from build123d import *

# Parameters (mm, degrees)
CROQUIS1_R              = 4.75
CROQUIS1_R_2            = 3.275
SALIENTE_EXTRUIR1_DEPTH = 4.25
CROQUIS3_R              = 4.85
CROQUIS3_R_2            = 2.1
SALIENTE_EXTRUIR2_DEPTH = 2
REDONDEO1_R             = 0.6
REDONDEO2_R             = 1
CHAFL_N1_SIZE           = 0.7
CHAFL_N2_SIZE           = 0.5


with BuildPart() as part:
    # Croquis1 → Saliente-Extruir1 (new body)
    with BuildSketch(Plane(origin=(0, 0, 0), x_dir=(1, 0, 0), z_dir=(0, 1, 0))):
        Circle(CROQUIS1_R)
        Circle(CROQUIS1_R_2, mode=Mode.SUBTRACT)
    extrude(amount=SALIENTE_EXTRUIR1_DEPTH)

    # Croquis2 → Revolución1 (revolve)
    with BuildSketch(Plane.XY):
        Polygon((-4.75, 4.25), (-4.85, 5.25), (-2.1, 5.25), (-2.1, 5.15), (-3.275, 4.25), align=None)
    revolve(axis=Axis((0, 0, 0), (0, 1, 0)))

    # Croquis3 → Saliente-Extruir2 (add)
    with BuildSketch(Plane(origin=(0, 5.25, 0), x_dir=(1, 0, 0), z_dir=(0, 1, 0))):
        Circle(CROQUIS3_R)
        Circle(CROQUIS3_R_2, mode=Mode.SUBTRACT)
    extrude(amount=SALIENTE_EXTRUIR2_DEPTH)

    # Redondeo1
    redondeo1_edges = [part.edges().sort_by_distance(p)[0] for p in [
        (-4.85, 7.25, 0),
    ]]
    fillet(redondeo1_edges, radius=REDONDEO1_R)

    # Redondeo2
    redondeo2_edges = [part.edges().sort_by_distance(p)[0] for p in [
        (2.1, 5.15, 0),
    ]]
    fillet(redondeo2_edges, radius=REDONDEO2_R)

    # Chaflán1
    chafl_n1_edges = [part.edges().sort_by_distance(p)[0] for p in [
        (-3.275, 0, 0),
    ]]
    chamfer(chafl_n1_edges, length=CHAFL_N1_SIZE)

    # Chaflán2
    chafl_n2_edges = [part.edges().sort_by_distance(p)[0] for p in [
        (-2.1, 7.25, 0),
    ]]
    chamfer(chafl_n2_edges, length=CHAFL_N2_SIZE)


solid = part.part
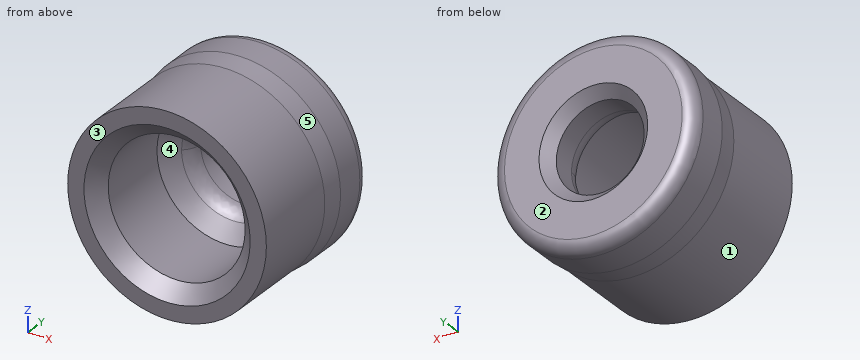
Geometry: final body of the model. Coordinates: model frame, mm. Face numbers are marked on the shaded views. A direction names the side the tool comes from. Round coordinates to 2 decimals unless told otherwise and drop trailing zeros. Loops run counter-clockwise (first coordinate to the right, second up) from the corner with the lowest first, then second, coordinate; pieces in that order, holes last. Notation, with made-up numbers: M 33.5,-31 L 38.5,-31 A20 ccw 38.5,-6 Z; hole C 45,22 d6. An arc over 180 degrees is marked long. One line per question, with ' | ' between items.
(1) Pull-direction query (X, two-part tool) for the marked faces 3, 4 and 5; classes: +X half, -X half, draft (parallel to the pull), parting line (faces both ways), or undercut.
Check result:
face 3: draft | face 4: undercut | face 5: parting line
(2) Cut plane A-A on y = 6.5. Return the cut outline in (x, z), plus the area to 3 significant figures.
Check result:
outline: C 0,0 d9.7; hole C 0,0 d4.2 | area: 60.0 mm2
(3) Access query for the marked faces 1 and 2. Directions: +Z, -Z, +X, -X, +Y, -Y. A direction counts if a zero-diameter tool reaches every point of the face in a straight line with its end or side. Return the directions, or none.
Check result:
face 1: -Y | face 2: +Z, -Z, +X, -X, +Y
(4) Cut plane B-B on y = 3.75. Return the cut outline in (x, z) (3 decimals).
Check result:
outline: C 0,0 d9.5; hole C 0,0 d6.55
(5) Contact query for flat-ended pins moving along their axis: P1, Ø3, axis at y = 1.5, z = 1, coming from the +X side; P2, Ø2, axis at x = 1, y = 2, coming from the +Z side; P3, Ø4, axis at x = 0.5, z = -1, coming from the +Y side. Output: stop coordinate, or through.
Check result:
P1: stops at x = 4.75 | P2: stops at z = 4.75 | P3: stops at y = 7.25
(6) Material intervals for line 1 along Z through (x, y) = (0, 6); line 2 along Z through (x, y) = (0, 2.25) (3 decimals), sorted ascending. Write a range as from..to.
Check result:
line 1: z = -4.85..-2.1, 2.1..4.85 | line 2: z = -4.75..-3.275, 3.275..4.75
